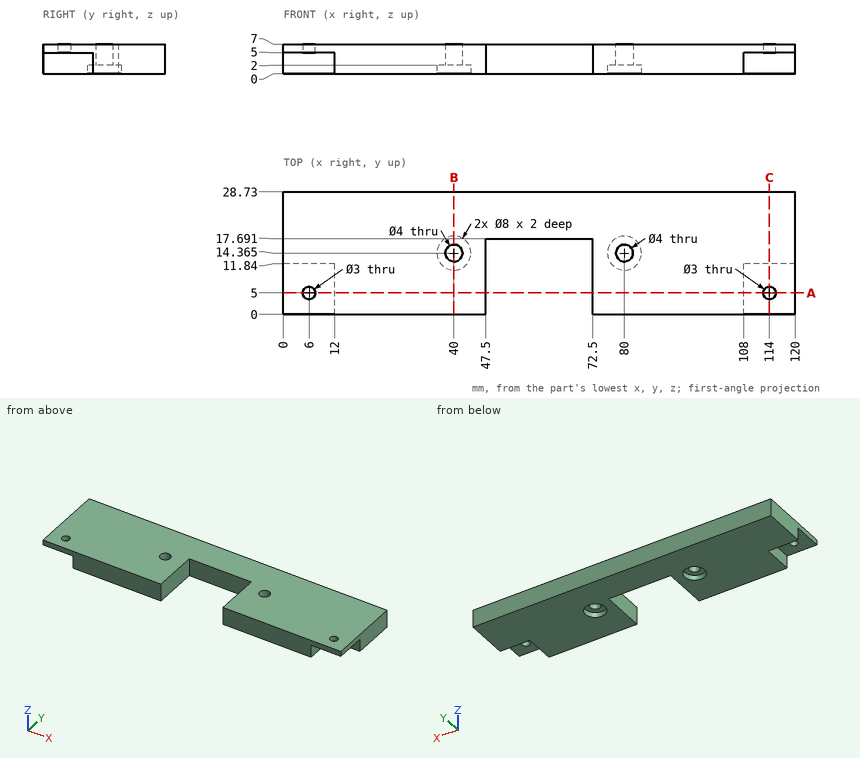
Geometry check sheet. Reference: drawing and pictorial views, mm from the part's lowest x, y, z. Give positions to 0.01 mm unless a question says otherwise; leave off trailing zeros. Order: outer loops, then holes, each group sorted by start corner. A loop starts at its lowest first (then second) coordinate and runs counter-clockwise, first axis right, second up. Notation, with made-up numbers: M -24.5,60.25 L -19.5,60.25 A9 cw -19.5,71.25 Z; hole C 48.25,-15.5 d8. An arc over 180 degrees is marked long. Answer as a JSON object with one key per item and string values. Group by question number.
1) Cross-section at B-B (x = 40). Enter the section's corners in (y, z) (1 decimal).
2) Scan lines: line 1 along X through (y, z) = (5, 6.05); line 2 along X through (y, z) = (7.5, 4); line 3 along X through (y, z) = (16, 5.5). Record each from-to range of solid material in increasing order. Write a range as [from, to].
3) Cross-section at A-A (y = 5). Enter the section's corners in (x, z).
4) Cross-section at C-C (x = 114). Enter the section's corners in (y, z), then the cut area to 3 significant figures.
5) Depth check by flat-ended pin: pin 1 Ø4 at (x, y) = (41, 13.5) entering from -Z; pin 2 Ø2 at (x, z) = (63.5, 5) entering from -Y; pin 3 Ø1 at (y, z) = (10.5, 3) entering from +X. Enter the tip coordinate at first touch or a pass-through.
Result sheet:
{
 "1": {"outline": "M 0,0 L 10.4,0 L 10.4,2 L 12.4,2 L 12.4,7 L 0,7 Z; M 16.4,2 L 18.4,2 L 18.4,0 L 28.7,0 L 28.7,7 L 16.4,7 Z"},
 "2": {"line 1": "x = [0, 4.5], [7.5, 47.5], [72.5, 112.5], [115.5, 120]", "line 2": "x = [12, 47.5], [72.5, 108]", "line 3": "x = [0, 38.85], [41.15, 47.5], [72.5, 78.85], [81.15, 120]"},
 "3": {"outline": "M 0,5 L 4.5,5 L 4.5,7 L 0,7 Z; M 7.5,5 L 12,5 L 12,0 L 47.5,0 L 47.5,7 L 7.5,7 Z; M 72.5,0 L 108,0 L 108,5 L 112.5,5 L 112.5,7 L 72.5,7 Z; M 115.5,5 L 120,5 L 120,7 L 115.5,7 Z"},
 "4": {"outline": "M 0,5 L 3.5,5 L 3.5,7 L 0,7 Z; M 6.5,5 L 11.84,5 L 11.84,0 L 28.73,0 L 28.73,7 L 6.5,7 Z", "area": "136 mm2"},
 "5": {"pin 1": "stops at z = 2", "pin 2": "stops at y = 17.69", "pin 3": "stops at x = 108"}
}
